Can you work these out from the model? Positions are in its coordinate system, mm. Face numbers are marked on the shaded views. A direction names the side the tool comes from. Give positions to 0.01 mm unless a question says otherwise; leave off trailing zeros. Order: outer loops, then holes, each group sorted by start corner. A loop starts at its lowest first (then second) coordinate and runs counter-clockwise, first axis right, second up. Notation, with made-up numbers: M 44.5,25.5 L 66.5,25.5 A20 ccw 66.5,41.5 Z; hole C -23,-9 d10. An arc over 180 degrees is marked long. One line per question, with ' | ' between items. Start each with the question number.
1) I'm going to push flat-ended pins straight in: pin 1 Ø2 at (x, z) = (-14.5, 5) entering from -Y; pin 2 Ø3.5 at (x, y) = (-19, 24) entering from +Z; pin 3 Ø1.5 at (y, z) = (-16, 6.5) entering from +X. Where does each tip first touch, or does it pass through?
2) If we section it at B-B, the plane z = 3: Please give me the cut outline in (x, y).
3) If we section it at C-C, the plane x = -2.5: Please give me the cut outline in (y, z), plus the area to 3 significant figures.
4) If we section it at D-D, the plane z = 9.75: Please give me the cut outline in (x, y), plus the area to 3 significant figures.
5) For the marked faces 1, 2, 3 and 4, which set-ups out of +Z, -Z, +X, -X, +Y, -Y let a thin tool reach every point of the face, with its end or its side?
6) Please list where these lines run through material, in increasing order: line 1 along Y through (x, z) = (7, 10.25); line 2 along Y through (x, z) = (-20.1, 0.8); line 3 along Y through (x, z) = (-35, 2). Write a range as [from, to].
7) Thinking about a two-plate mould opening in Y: for the marked faces 5, 6, 7 and 8, which applies, +Y half, -Y half, draft (parallel to the pull), parting line (faces both ways), or undercut?
8) If we section it at A-A, the plane y = 24: Please give me the cut outline in (x, z), plus the area to 3 significant figures.
```python
from build123d import *

# Parameters (mm, degrees)
F0_R     = 1.6
F0_W     = 38
F0_H     = 2
F0_W_2   = 7
F0_H_2   = 5
F0_W_3   = 5
F0_H_3   = 7
F0_W_4   = 47.5
F1_DEPTH = 1.6
F0_W_5   = 6.2
F0_H_4   = 12
F0_W_6   = 8.8
F0_W_7   = 1.8
F0_H_5   = 8.9
F0_W_8   = 11.2
F2_DEPTH = 12.6
F3_DEPTH = 10.6
F4_R     = 3.175
F5_DEPTH = 12.7


with BuildPart() as f1:
    # F0 (on Top) → F1 (new body)
    with BuildSketch(Plane.XY):
        Polygon((31.5, 13.5), (31.5, 26.5), (-34, 26.5), (-34, 16.9), (-25.2, 16.9), (-25.2, 4.9), (-34, 4.9), (-34, -14.3), (-22.8, -14.3), (-22.8, -23.2), (-34, -23.2), (-34, -26.5), (31.5, -26.5), (31.5, -24.5), (34, -21.5), (34, 10.5), align=None)
        with Locations((-20.1, -24.2)):
            Circle(F0_R, mode=Mode.SUBTRACT)
        with Locations((11.5, -23.96)):
            Rectangle(F0_W, F0_H, mode=Mode.SUBTRACT)
        with Locations((31.5, -19.5)):
            Circle(F0_R, mode=Mode.SUBTRACT)
        with Locations((-16, 19.3)):
            Rectangle(F0_W_2, F0_H_2, mode=Mode.SUBTRACT)
        with Locations((-19, 24)):
            Circle(F0_R, mode=Mode.SUBTRACT)
        with Locations((30.5, 1.1)):
            Rectangle(F0_W_3, F0_H_3, mode=Mode.SUBTRACT)
        with Locations((31.5, 8.5)):
            Circle(F0_R, mode=Mode.SUBTRACT)
        with Locations((6.75, 24)):
            Rectangle(F0_W_4, F0_H, mode=Mode.SUBTRACT)
    extrude(amount=F1_DEPTH)

    # F0 (on Top) → F2 (join)
    with BuildSketch(Plane.XY):
        with Locations((-37.1, 10.9)):
            Rectangle(F0_W_5, F0_H_4)
        with Locations((-29.6, 10.9)):
            Rectangle(F0_W_6, F0_H_4)
        with Locations((-34.9, -18.75)):
            Rectangle(F0_W_7, F0_H_5)
        with Locations((-28.4, -18.75)):
            Rectangle(F0_W_8, F0_H_5)
    extrude(amount=F2_DEPTH)

    # F0 (on Top) → F3 (join)
    with BuildSketch(Plane.XY):
        with Locations((6.75, 24)):
            Rectangle(F0_W_4, F0_H)
        with Locations((11.5, -23.96)):
            Rectangle(F0_W, F0_H)
        with Locations((-16, 19.3)):
            Rectangle(F0_W_2, F0_H_2)
        with Locations((30.5, 1.1)):
            Rectangle(F0_W_3, F0_H_3)
    extrude(amount=F3_DEPTH)

    # F4 (on face) → F5 (cut)
    with BuildSketch(Plane(origin=(-35.8, 0, 0), x_dir=(0, -1, 0), z_dir=(-1, 0, 0))):
        with Locations((18.745, 7.823)):
            Circle(F4_R)
    extrude(amount=-F5_DEPTH, mode=Mode.SUBTRACT)


solid = f1.part
```
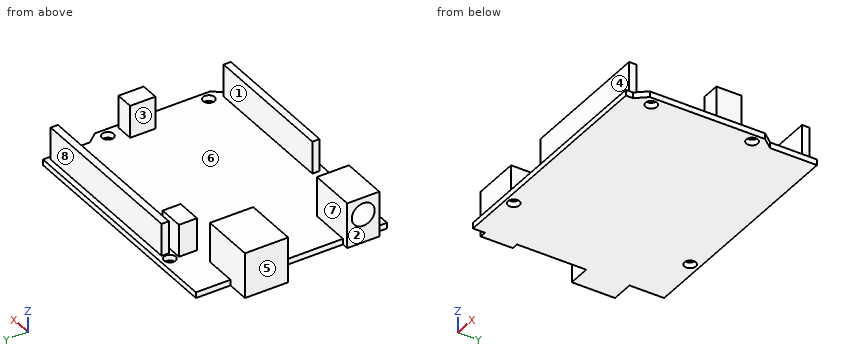
Results found:
1) pin 1: stops at y = 16.8 | pin 2: stops at z = 1.6 | pin 3: stops at x = -22.8
2) outline: M -40.2,4.9 L -25.2,4.9 L -25.2,16.9 L -40.2,16.9 Z; M -35.8,-23.2 L -22.8,-23.2 L -22.8,-14.3 L -35.8,-14.3 Z; M -19.5,16.8 L -12.5,16.8 L -12.5,21.8 L -19.5,21.8 Z; M -17,23 L 30.5,23 L 30.5,25 L -17,25 Z; M -7.5,-24.96 L 30.5,-24.96 L 30.5,-22.96 L -7.5,-22.96 Z; M 28,-2.4 L 33,-2.4 L 33,4.6 L 28,4.6 Z
3) outline: M -26.5,0 L 26.5,0 L 26.5,1.6 L 25,1.6 L 25,10.6 L 23,10.6 L 23,1.6 L -22.96,1.6 L -22.96,10.6 L -24.96,10.6 L -24.96,1.6 L -26.5,1.6 Z | area: 121 mm²
4) outline: M -40.2,4.9 L -25.2,4.9 L -25.2,16.9 L -40.2,16.9 Z; M -35.8,-23.2 L -22.8,-23.2 L -22.8,-14.3 L -35.8,-14.3 L -35.8,-16.22 L -23.1,-16.22 L -23.1,-21.27 L -35.8,-21.27 Z; M -19.5,16.8 L -12.5,16.8 L -12.5,21.8 L -19.5,21.8 Z; M -17,23 L 30.5,23 L 30.5,25 L -17,25 Z; M -7.5,-24.96 L 30.5,-24.96 L 30.5,-22.96 L -7.5,-22.96 Z; M 28,-2.4 L 33,-2.4 L 33,4.6 L 28,4.6 Z | area: 473 mm²
5) face 1: +Z, +X | face 2: +Z, -Z, -X, -Y | face 3: +Z, -X | face 4: +Z, +X, -X, -Y
6) line 1: y = [-24.96, -22.96], [23, 25] | line 2: y = [-26.5, -25.8], [-22.6, 22.84], [25.16, 26.5] | line 3: y = [-23.2, -14.3], [4.9, 16.9]
7) face 5: draft | face 6: undercut | face 7: undercut | face 8: +Y half
8) outline: M -34,0 L -20.6,0 L -20.6,1.6 L -34,1.6 Z; M -17.4,0 L 31.5,0 L 31.5,1.6 L 30.5,1.6 L 30.5,10.6 L -17,10.6 L -17,1.6 L -17.4,1.6 Z | area: 527 mm²
